Geometry check sheet. Reference: the model listing, model coordinates, mm. Face numbers are marked on the shaded views. A direction names the side the tool comes from. Round coordinates to 2 decimals unless told otherwise and drop trailing zeros. Loops run counter-clockwise (first coordinate to the right, second up) from the corner with the lowest first, then second, coordinate; pieces in that order, holes last. Notation, with made-up numbers: (73, 52) -> (102, 52) arc R15 cw to (102, 77) -> close; hole circle Ø8 at (66, 55). An arc over 180 degrees is marked (long way). Use a Markdown table: item, result. Add a question column.
Q1. Material ranges on L1, parallel to Y at x = 0, z = 9; L2, parallel to Z at x = 90, y = -1; L3, parallel to Y at x = -4.5, z = -21, recorded low to high.
Q2. Set-up check for the marked faces 1, 2 and 3: record each of +Z, -Z, +X, -X, +Y, -Y from which the full face is reachable in a straight line by a thin tool's end or side.
Q3. Sectioned sample at A-A, the plane x = 0. Enter the section's corners in (y, z).
Q4. Release check for a two-part mould opening along X. For the marked faces 4, 5, 6 and 7 record: released by +X, released by -X, zero draft, split by the parting line, or undercut.
Q5. Gauge pin test, flat ends, axial feed: P1, Ø10, axis at x = 93.5, y = -6.5, coming from the +Z side; P2, Ø1, axis at x = -54.5, z = 7.5, coming from the -Y side; P3, Ø8, axis at y = -17, z = -1.5, coming from the -X side. Record the tip position at first contact, or that the pin passes through.
Q6. Sectioned sample at B-B, the plane y = 23. Enter the section's corners in (x, z), then the cut area to 3 significant figures.
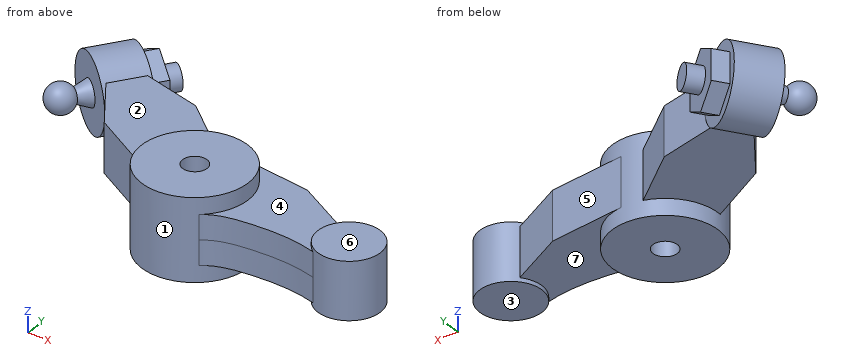
```python
from build123d import *

# Parameters (mm, degrees)
SKETCH1_R           = 33.02
SKETCH1_R_2         = 7.62
BOSS_EXTRUDE1_DEPTH = 25.4
SKETCH1_3_R         = 19.3675
BOSS_EXTRUDE2_DEPTH = 17.78
BOSS_EXTRUDE3_DEPTH = 15.24
BOSS_EXTRUDE4_DEPTH = 15.24
BOSS_EXTRUDE5_DEPTH = 10.16
SKETCH8_R           = 7.62
BOSS_EXTRUDE6_DEPTH = 10.16


with BuildPart() as part:
    # Sketch1 → Boss-Extrude1 (new, symmetric)
    with BuildSketch(Plane.XY):
        Circle(SKETCH1_R)
        Circle(SKETCH1_R_2, mode=Mode.SUBTRACT)
    extrude(amount=BOSS_EXTRUDE1_DEPTH, both=True)



with BuildPart() as body_2:
    # Sketch1_3 → Boss-Extrude2 (new, symmetric)
    with BuildSketch(Plane.XY):
        with Locations((101.092, -6.347255181)):
            Circle(SKETCH1_3_R)
    extrude(amount=BOSS_EXTRUDE2_DEPTH, both=True)


with BuildPart() as part_1:
    add(part.part)

    add(body_2.part)  # Boss-Extrude3 merges body 2
    # Sketch1_4 → Boss-Extrude3 (add, symmetric)
    with BuildSketch(Plane.XY):
        with BuildLine():
            ThreePointArc((89.316955097, -21.724133075), (81.821344439, -8.281651859), (86.495604602, 6.382446214))
            Line((86.495604602, 6.382446214), (51.99535192, 25.990827948))
            Line((51.99535192, 25.990827948), (4.626759051, 32.694242623))
            ThreePointArc((4.626759051, 32.694242623), (24.930864244, 21.651152581), (33.02, 0))
            ThreePointArc((33.02, 0), (29.814370972, -14.19238118), (20.819898028, -25.62912886))
            add(Edge.make_bspline(
                [(89.316955097, -21.724133075), (75.276461203, -17.426169931), (52.836610599, -16.671014881), (28.008203074, -19.789688164), (20.819898028, -25.62912886)],
                knots=[0, 0, 0, 0, 0.609501507, 1, 1, 1, 1], degree=3))
        make_face()
    extrude(amount=BOSS_EXTRUDE3_DEPTH, both=True)

    # Sketch1_5 → Boss-Extrude4 (add, symmetric)
    with BuildSketch(Plane.XY):
        with BuildLine():
            ThreePointArc((-32.953500531, -2.094565059), (-26.892130639, 19.160733538), (-8.781498221, 31.830892055))
            Line((-8.781498221, 31.830892055), (-42.262603979, 60.502117005))
            Line((-42.262603979, 60.502117005), (-86.872548051, 72.422885384))
            Line((-86.872548051, 72.422885384), (-96.821390465, 58.459663706))
            Line((-96.821390465, 58.459663706), (-70.986413412, 20.188188826))
            Line((-70.986413412, 20.188188826), (-32.953500531, -2.094565059))
        make_face()
    extrude(amount=BOSS_EXTRUDE4_DEPTH, both=True)



with BuildPart() as body_2_2:
    # Sketch5 → Revolve2 (revolve)
    with BuildSketch(Plane.XY, mode=Mode.PRIVATE) as revolve2_sk:
        with BuildLine():
            Line((-96.821390465, 58.459663706), (-86.20929189, 73.353766829))
            Line((-86.20929189, 73.353766829), (-94.483793625, 79.249377149))
            Line((-94.483793625, 79.249377149), (-122.603936438, 39.782696366))
            ThreePointArc((-122.603936438, 39.782696366), (-111.841735812, 40.121260824), (-109.299895081, 50.584464631))
            Line((-109.299895081, 50.584464631), (-96.821390465, 58.459663706))
        make_face()
    revolve(revolve2_sk.sketch.rotate(Axis((-94.483793625, 79.249377149, 0), (-0.5802766062403011, -0.8144194621018328, 0)), 180), axis=Axis((-94.483793625, 79.249377149, 0), (-0.5802766062403011, -0.8144194621018328, 0)))


with BuildPart() as part_2:
    add(part_1.part)

    add(body_2_2.part)  # Revolve4 merges body 2 2
    # Sketch6 → Revolve4 (revolve)
    with BuildSketch(Plane.XY):
        Polygon((-108.193400918, 60.007913893), (-92.275253056, 82.349068577), (-111.099744503, 95.761582054), (-127.017892365, 73.42042737), align=None)
    revolve(axis=Axis((-94.483793625, 79.249377149, 0), (-0.5802766062403006, -0.8144194621018331, 0)))

    # Sketch7 → Boss-Extrude5 (add)
    with BuildSketch(Plane(origin=(7.846217937, 11.012183713, 0), x_dir=(0.814419462101833, -0.5802766062403008, 0), z_dir=(0.5802766062403008, 0.8144194621018331, 0))):
        Polygon((-106.426, -9.532052944), (-106.426, 9.532052944), (-122.936, 19.064105889), (-139.446, 9.532052944), (-139.446, -9.532052944), (-122.936, -19.064105889), align=None)
    extrude(amount=BOSS_EXTRUDE5_DEPTH)

    # Sketch8 → Boss-Extrude6 (add)
    with BuildSketch(Plane(origin=(13.741828257, 19.286685448, 0), x_dir=(0.814419462101833, -0.5802766062403008, 0), z_dir=(0.5802766062403008, 0.8144194621018331, 0))):
        with Locations(Location((-122.936, 0, 0), (0, 0, 180))):
            Circle(SKETCH8_R)
    extrude(amount=BOSS_EXTRUDE6_DEPTH)


solid = part_2.part
```
Values:
| question | item | result |
|---|---|---|
| 1 | L1 | -33.02 to -7.62, 7.62 to 33.02 |
| 1 | L2 | -17.78 to 17.78 |
| 1 | L3 | -32.71 to -6.15, 6.15 to 32.71 |
| 2 | face 1 | none |
| 2 | face 2 | +Z |
| 2 | face 3 | -Z, +X, +Y, -Y |
| 3 | outline | (-33.02, -25.4) -> (-7.62, -25.4) -> (-7.62, 25.4) -> (-33.02, 25.4) -> close; (7.62, -25.4) -> (33.02, -25.4) -> (33.02, 25.4) -> (7.62, 25.4) -> close |
| 4 | face 4 | undercut |
| 4 | face 5 | released by +X |
| 4 | face 6 | zero draft |
| 4 | face 7 | undercut |
| 5 | P1 | z = 17.78 |
| 5 | P2 | y = 10.24 |
| 5 | P3 | x = -30.35 |
| 6 | outline | (-72.88, -15.24) -> (-23.69, -15.24) -> (-23.69, -25.4) -> (23.69, -25.4) -> (23.69, -15.24) -> (57.26, -15.24) -> (57.26, 15.24) -> (23.69, 15.24) -> (23.69, 25.4) -> (-23.69, 25.4) -> (-23.69, 15.24) -> (-72.88, 15.24) -> close |
| 6 | area | 4,930 mm^2 |
